```python
from build123d import *

# Parameters (mm, degrees)
SKETCH1_R           = 2.6375
BOSS_EXTRUDE1_DEPTH = 4


with BuildPart() as part:
    # Sketch1 → Boss-Extrude1 (new body)
    with BuildSketch(Plane(origin=(0, 4, 0), x_dir=(1, 0, 0), z_dir=(0, 1, 0))):
        with BuildLine():
            Line((80.422342857, 54.050517259), (76.853623233, 60.632336961))
            ThreePointArc((76.853623233, 60.632336961), (76.491061204, 62.093363418), (76.883808504, 63.546566463))
            ThreePointArc((76.883808504, 63.546566463), (76.887801931, 63.553594024), (76.891783993, 63.560628031))
            ThreePointArc((76.891783993, 63.560628031), (77.252393533, 65.441834253), (76.401227258, 67.157786484))
            Line((76.401227258, 67.157786484), (74.710106586, 68.848907157))
            ThreePointArc((74.710106586, 68.848907157), (73.793959033, 69.474868842), (72.712949954, 69.725016274))
            Line((72.712949954, 69.725016274), (69.341583584, 69.864669723))
            Line((69.341583584, 69.864669723), (58.04793187, 69.864669723))
            ThreePointArc((58.04793187, 69.864669723), (56.905384642, 70.210123831), (56.115987655, 71.105447853))
            Line((56.115987655, 71.105447853), (45.913475043, 90.139986308))
            ThreePointArc((45.913475043, 90.139986308), (45.078544808, 92.769966676), (45.661998303, 95.466907026))
            Line((45.661998303, 95.466907026), (47.984386737, 99.06049755))
            ThreePointArc((47.984386737, 99.06049755), (49.146460916, 100.107430356), (50.677561656, 100.427141511))
            ThreePointArc((50.677561656, 100.427141511), (55.107636105, 111.997063252), (44.809847991, 105.109087593))
            ThreePointArc((44.809847991, 105.109087593), (44.89620964, 103.838561027), (44.447757125, 102.646677462))
            Line((44.447757125, 102.646677462), (40.917682236, 97.184351056))
            ThreePointArc((40.917682236, 97.184351056), (40.000914232, 93.684113367), (40.729811239, 90.139986308))
            Line((40.729811239, 90.139986308), (52.448751423, 68.276291936))
            ThreePointArc((52.448751423, 68.276291936), (53.733769558, 66.46917356), (55.737555004, 65.519546097))
            Line((55.737555004, 65.519546097), (64.043852088, 65.068697747))
            Line((64.043852088, 65.068697747), (65.737001521, 65.002354827))
            ThreePointArc((65.737001521, 65.002354827), (67.167212394, 64.574619561), (68.214209712, 63.510543803))
            ThreePointArc((68.214209712, 63.510543803), (69.182612076, 62.314016036), (70.4690978, 61.468772687))
            ThreePointArc((70.4690978, 61.468772687), (71.304443417, 60.902477838), (71.904734595, 60.091217919))
            Line((71.904734595, 60.091217919), (76.886572185, 50.235843556))
            ThreePointArc((76.886572185, 50.235843556), (77.175676431, 49.329685255), (77.166582589, 48.378569367))
            ThreePointArc((77.166582589, 48.378569367), (85.084005766, 43.530139369), (82.698094563, 52.502334805))
            ThreePointArc((82.698094563, 52.502334805), (81.37218956, 53.000032473), (80.422342857, 54.050517259))
        make_face()
        with Locations((51.053576092, 106.916256485)):
            Circle(SKETCH1_R, mode=Mode.SUBTRACT)
        with Locations((82.095552315, 47.538773298)):
            Circle(SKETCH1_R, mode=Mode.SUBTRACT)
        with Locations((72.538655529, 66.020358214)):
            Circle(SKETCH1_R, mode=Mode.SUBTRACT)
    extrude(amount=-BOSS_EXTRUDE1_DEPTH)


solid = part.part
```
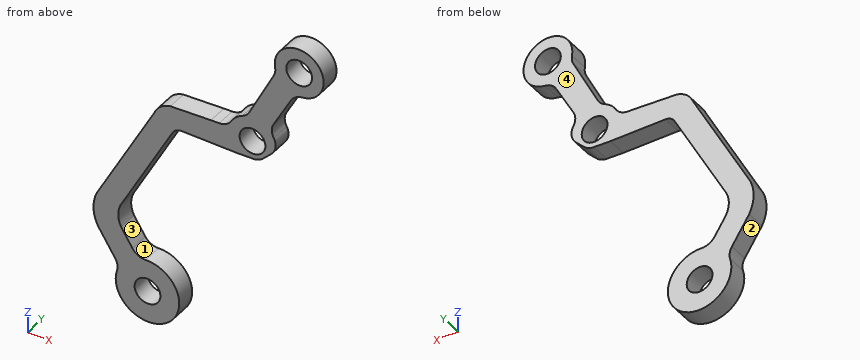
Geometry check sheet. Reference: the model listing, model coordinates, mm. Face numbers are marked on the shaded views. Coordinates: 2 decimals unless noted, no trailing zeros. Order: outer loops, then holes, each group sorted by start corner. A loop starts at its lowest first (then second) coordinate and runs counter-clockwise, first axis right, second up. Notation, with made-up numbers: (-1.75, 40) - (26.25, 40) arc R27 ccw to (26.25, 60) - close; hole circle Ø11 at (-18, 70). An arc over 180 degrees is marked (long way). Answer in a Markdown table with one row per item. Add a question column.
1. Draft check along Z on the marked faces 1, 2, 3 and 4. Enter one of: +Z half, -Z half, draft (parallel to the pull), parting line (faces both ways), or undercut.
2. Section check C-C (x = 67). Enter the section's corners in (y, z), plus the area to 3 significant figures.
3. Material ranges on L1, parallel to Z at x = 49.5, y = 3.85; L2, parallel to X at y = 2.35, z = -106.5; L3, parallel to Z at x = 65.5, y = 0.95, recorded low to high. Write a range as [from, to].
4. Section check A-A (y = 3). Give the number of separate pieces and of enclosed holes in the cut face, plus the area to 3 significant figures.
5. Section check B-B (z = -98). Enter the section's corners in (x, y), plus the area to 3 significant figures.
6. Gauge pin test, flat ends, axial feed: pin 1 Ø2 at (y, z) = (3.5, -55.5) entering from -X; pin 2 Ø6 at (x, z) = (72.54, -66.02) entering from +Y. Record the tip position at first contact, or that the pin passes through.
Data:
| question | item | result |
|---|---|---|
| 1 | face 1 | undercut |
| 1 | face 2 | -Z half |
| 1 | face 3 | undercut |
| 1 | face 4 | draft |
| 2 | outline | (0, -69.86) - (4, -69.86) - (4, -64.67) - (0, -64.67) - close |
| 2 | area | 20.8 mm² |
| 3 | L1 | z = [-113.23, -109.05], [-104.78, -100.26], [-83.45, -73.78] |
| 3 | L2 | x = [44.57, 48.45], [53.66, 57.54] |
| 3 | L3 | z = [-69.86, -65.01] |
| 4 | separate pieces | 1 |
| 4 | enclosed holes | 3 |
| 4 | area | 510 mm² |
| 5 | outline | (41.44, 0) - (47.3, 0) - (47.3, 4) - (41.44, 4) - close |
| 5 | area | 23.4 mm² |
| 6 | pin 1 | stops at x = 73.72 |
| 6 | pin 2 | stops at y = 4 |
